CAD build for the part. Positions are in the model's coordinates, mm. A direction names the side the tool comes from. Coordinates: 2 decimals unless noted, no trailing zeros. Write each loop counter-clockwise with the first axis right and the second up, starting at its lowest first coordinate (ties: lowest second). Pieces come first, ordered by that corner, then holes. Notation, with made-up numbers: (3.5, 72) - (18.5, 72) arc R15 ccw to (18.5, 77) - close; hole circle Ø9 at (27, 72). An arc over 180 degrees is marked (long way). Answer in a Markdown table with one row per item. Add a question column.
Q1. Band-saw the part on C-C (z = 11). List the corners of the cut face in (x, y).
Q2. Band-saw the part on A-A (x = 0). List the corners of the cut face in (y, z).
Q3. Drill centre lines: line 1 along Z through (x, y) = (0.5, -1.75); line 2 along Z through (x, y) = (2, 0.75); line 3 along X through (y, z) = (0, 24.5). Where is each one in solid material? Low to high. Write a range as from..to.
Q4. Pin check, flat tips, straight feed: pin 1 (3 mm diameter, centred on y = -2, z = 17.5, fed in from +X); pin 2 (1 mm diameter, centred on x = -2, y = 2, fed in from -Z); pin 3 (4 mm diameter, centred on x = -1.5, z = 22, fed in from -Y). Stop position of each tip, or through.
Q5. 3-axis set-ups, long thin cutter, end or side, ignore diameter. For faces 1 (the flat face through (-2, -2, 13)), 2 (the cylindrical face through (-3.233, -1.341, 13.507)), 3 (the cylindrical face through (0, -1, 32)): which of +Z, -Z, +X, -X, +Y, -Y reach the whole face in a straight line?
Q6. Band-saw the part on D-D (x = 1.5). List the corners of the cut face in (y, z).
```python
from build123d import *

# Parameters (mm, degrees)
EXTRUDE_START   = 3.386462
SKETCH_1_R      = 2
EXTRUDE_1_DEPTH = 27.013538
SKETCH_2_R      = 1
EXTRUDE_2_DEPTH = 2.6
SKETCH_4_R      = 1
EXTRUDE_3_DEPTH = 2.6
EXTRUDE_START_2 = -10.613538
SKETCH_6_R      = 3.5
EXTRUDE_5_DEPTH = 1


with BuildPart() as part:
    # Эскиз1 → Бобышка-Вытянуть1 (new body)
    with BuildSketch(Plane.XY.offset(EXTRUDE_START)):
        Circle(SKETCH_1_R)
    extrude(amount=EXTRUDE_1_DEPTH)

    # Эскиз2 → Бобышка-Вытянуть2 (add)
    with BuildSketch(Plane.XY.offset(30.4)):
        Circle(SKETCH_2_R)
    extrude(amount=EXTRUDE_2_DEPTH)

    # Эскиз4 → Бобышка-Вытянуть3 (add)
    with BuildSketch(Plane(origin=(0, 0, 3.386462289), x_dir=(-1, 0, 0), z_dir=(0, 0, -1))):
        Circle(SKETCH_4_R)
    extrude(amount=EXTRUDE_3_DEPTH)

    # Эскиз6 → Бобышка-Вытянуть5 (add)
    with BuildSketch(Plane(origin=(0, 0, 3.386462289), x_dir=(-1, 0, 0), z_dir=(0, 0, -1)).offset(EXTRUDE_START_2)):
        Circle(SKETCH_6_R)
    extrude(amount=EXTRUDE_5_DEPTH)


solid = part.part
```
Checked values:
| question | item | result |
|---|---|---|
| 1 | outline | circle Ø4 at (0, 0) |
| 2 | outline | (-3.5, 13) - (-2, 13) - (-2, 3.39) - (-1, 3.39) - (-1, 0.79) - (1, 0.79) - (1, 3.39) - (2, 3.39) - (2, 13) - (3.5, 13) - (3.5, 14) - (2, 14) - (2, 30.4) - (1, 30.4) - (1, 33) - (-1, 33) - (-1, 30.4) - (-2, 30.4) - (-2, 14) - (-3.5, 14) - close |
| 3 | line 1 | z = 3.39..30.4 |
| 3 | line 2 | z = 13..14 |
| 3 | line 3 | x = -2..2 |
| 4 | pin 1 | stops at x = 1.94 |
| 4 | pin 2 | stops at z = 13 |
| 4 | pin 3 | stops at y = -2 |
| 5 | face 1 | -Z |
| 5 | face 2 | +Z, -Z |
| 5 | face 3 | +Z |
| 6 | outline | (-3.16, 13) - (-1.32, 13) - (-1.32, 3.39) - (1.32, 3.39) - (1.32, 13) - (3.16, 13) - (3.16, 14) - (1.32, 14) - (1.32, 30.4) - (-1.32, 30.4) - (-1.32, 14) - (-3.16, 14) - close |
